Source: CAD feature listing. Evaluate the final solid. Frame: model axes, mm. Face numbers are marked on the shaded views. A direction names the side the tool comes from. Give positions to 0.01 mm unless a question says otherwise; leave off trailing zeros. Order: outer loops, then holes, each group sorted by start corner. A loop starts at its lowest first (then second) coordinate and runs counter-clockwise, first axis right, second up. Notation, with made-up numbers: M 25.5,85 L 65.5,85 A25 cw 65.5,103 Z; hole C 52.5,-29.75 d9. An arc over 180 degrees is marked long. Answer in a Markdown table with one row per item. Add a question column.
(1) Set-up query: the marked faces 1 and 2. Return all of +Z, -Z, +X, -X, +Y, -Y with unobstructed straight access to the full face (end or side cutting, diameter ignored); none if empty.
(2) Section query A-A, the plane x = 0. Return loops of the section in (y, z), plus the area to 3 significant figures.
(3) Section query C-C, the plane z = 7.5. Return loops of the section in (x, y), plus the area to 3 significant figures.
(4) Pin query (flat end, axial travel): P1, Ø1.5, axis at y = -36.5, z = 6.5, coming from the -X side; P2, Ø3, axis at y = -42.5, z = 3, coming from the +X side; P3, Ø2, axis at y = 41, z = 6, coming from the -X side. Return the tip coordinate at first contact, or that it passes through.
(5) Section query D-D, the plane x = -80. Return loops of the section in (y, z), plus the area to 3 significant figures.
(6) Material intervals for line 1 along Y through (x, z) = (0, 1.45); line 2 along Z through (x, y) = (-79.5, -27); line 3 along Y through (x, z) = (36, 4.5), sorted ascending.
from build123d import *

# Parameters (mm, degrees)
F0_R     = 100
F1_DEPTH = 3
F2_R     = 55
F3_DEPTH = 25
F4_R     = 57
F4_R_2   = 55
F5_DEPTH = 10


with BuildPart() as f1:
    # F0 (on Top) → F1 (new body)
    with BuildSketch(Plane.XY):
        Circle(F0_R)
    extrude(amount=F1_DEPTH)

    # F2 (on face) → F3 (cut)
    with BuildSketch(Plane.XY.offset(3)):
        Circle(F2_R)
    extrude(amount=-F3_DEPTH, mode=Mode.SUBTRACT)

    # F4 (on face) → F5 (join)
    with BuildSketch(Plane.XY.offset(3)):
        Circle(F4_R)
        Circle(F4_R_2, mode=Mode.SUBTRACT)
    extrude(amount=F5_DEPTH)


solid = f1.part
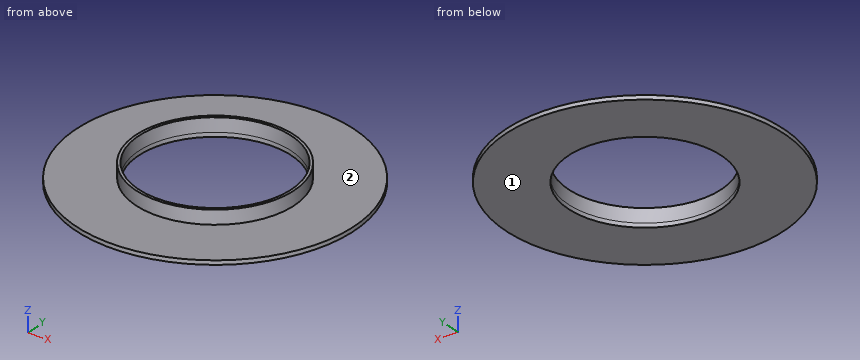
Values follow:
| question | item | result |
|---|---|---|
| 1 | face 1 | -Z, +X, -X, +Y, -Y |
| 1 | face 2 | +Z |
| 2 | outline | M -100,0 L -55,0 L -55,13 L -57,13 L -57,3 L -100,3 Z; M 55,0 L 100,0 L 100,3 L 57,3 L 57,13 L 55,13 Z |
| 2 | area | 310 mm² |
| 3 | outline | C 0,0 d114; hole C 0,0 d110 |
| 3 | area | 704 mm² |
| 4 | P1 | stops at x = -44.4 |
| 4 | P2 | stops at x = 91.21 |
| 4 | P3 | stops at x = -40.61 |
| 5 | outline | M -60,0 L 60,0 L 60,3 L -60,3 Z |
| 5 | area | 360 mm² |
| 6 | line 1 | y = -100 to -55, 55 to 100 |
| 6 | line 2 | z = 0 to 3 |
| 6 | line 3 | y = -44.19 to -41.58, 41.58 to 44.19 |
